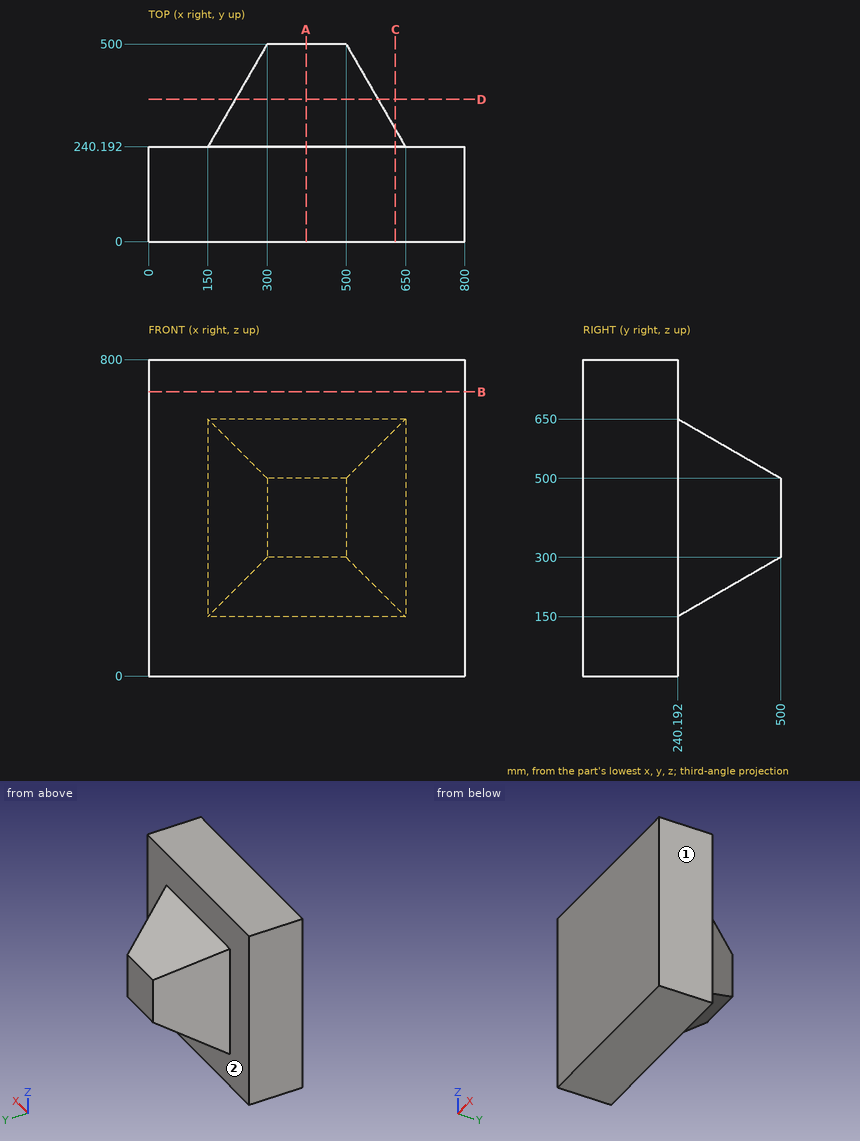
For this review, use the dimensioned drawing (mm, ordinates from the lowest corner) and the shaded views. A direction names the side the tool comes from. Give positions to 0.01 mm unless a question says otherwise; leave off trailing zeros. Write each loop counter-clockwise with the first axis right and the second up, starting at its lowest first coordinate (ties: lowest second). Pieces come first, ordered by that corner, then holes. Notation, with made-up numbers: M -36.75,-36.75 L -13.75,-36.75 A15 cw -13.75,-22.75 Z; hole C 41,52.25 d9. An arc over 180 degrees is marked long. Answer as a JSON object with one key per item and string values. Group by question number.
1) Tool access review of the marked faces 1 and 2: name each direction out of +Z, -Z, +X, -X, +Y, -Y from which nothing blocks a thin tool from reaching the whole face with its end or side.
2) We need section B-B (z = 718.5). Give the boundary of the cut face in (x, y), and give its area (3 significant figures).
3) Clearance check with flat-ended pins moving along their axes: pin 1 Ø2 at (x, y) = (338, 334.5) entering from +Z; pin 2 Ø5 at (x, y) = (556.5, 341) entering from -Z. State where each tip first meets the part, or that it passes through.
4) We need section D-D (y = 360). Give the boundary of the cut face in (x, z), and give its area (3 significant figures).
5) We need section A-A (x = 398.5). Give the boundary of the cut face in (y, z).
6) For line 1 along Y through (x, z) = (121, 317); line 2 along X through (y, z) = (450.5, 288); line 3 along Z through (x, y) = (374.5, 302) (1 decimal), list the stretches that pass through material, from the lowest coordinate up.
7) We need section C-C (x = 624.5). Give the boundary of the cut face in (y, z), and give its area (3 significant figures).
Answer key:
{
 "1": {"face 1": "+Z, -Z, +X, +Y, -Y", "face 2": "+Y"},
 "2": {"outline": "M 0,0 L 800,0 L 800,240.19 L 0,240.19 Z", "area": "192,000 mm²"},
 "3": {"pin 1": "stops at z = 596.13", "pin 2": "stops at z = 206.76"},
 "4": {"outline": "M 219.17,219.17 L 580.83,219.17 L 580.83,580.83 L 219.17,580.83 Z", "area": "131,000 mm²"},
 "5": {"outline": "M 0,0 L 240.19,0 L 240.19,150 L 500,300 L 500,500 L 240.19,650 L 240.19,800 L 0,800 Z"},
 "6": {"line 1": "y = 0 to 240.19", "line 2": "x = 271.42 to 528.58", "line 3": "z = 185.7 to 614.3"},
 "7": {"outline": "M 0,0 L 240.19,0 L 240.19,150 L 284.36,175.5 L 284.36,624.5 L 240.19,650 L 240.19,800 L 0,800 Z", "area": "213,000 mm²"}
}
